Design review of the part built by this model. Coordinates are the model's own, in mm. A direction names the side the tool comes from. Give positions to 0.01 mm unless a question says otherwise; leave off trailing zeros. Order: outer loops, then holes, each group sorted by start corner. A loop starts at its lowest first (then second) coordinate and runs counter-clockwise, first axis right, second up. Notation, with made-up numbers: (56.25, 20) - (64.25, 20) arc R19 ccw to (64.25, 28) - close; hole circle Ø3 at (-12, 87). An arc over 180 degrees is marked (long way). Write each question's results on one line, items separated by ' | '. Start each with the question number.
```python
from build123d import *

# Parameters (mm, degrees)
F0_W        = 29.464
F0_H        = 43.434
F1_DEPTH    = 25.4
F2_T1_DEPTH = 50.8
F3_R        = 5.08


# Not quite as in the source:
# - a fillet or chamfer that OpenCascade refuses, or shapes differently, is made with other operations: its cross-section is extruded or revolved along the edge and cut away or added


with BuildPart() as f1:
    # F0 (on Top) → F1 (new body)
    with BuildSketch(Plane.XY):
        Polygon((25.527, -26.797), (25.527, 26.797), (-25.527, 26.797), (-25.527, 0), (-20.447, 0), (-20.447, 21.717), (-14.097, 21.717), (-14.097, -26.797), align=None)
        with Locations((5.715, 0)):
            Rectangle(F0_W, F0_H, mode=Mode.SUBTRACT)
    extrude(amount=F1_DEPTH)

    # F2: fillet of radius 5.08 on 6 edges, made by hand

    # F2_s2 → F2_t1 (cut)
    with BuildSketch(Plane.XY.offset(-12.7)):
        with BuildLine():
            ThreePointArc((-20.447, 26.797), (-24.0391024484, 25.3091024484), (-25.527, 21.717))
            Line((-25.527, 21.717), (-25.527, 26.797))
            Line((-25.527, 26.797), (-20.447, 26.797))
        make_face()
        with BuildLine():
            ThreePointArc((25.527, 21.717), (24.0391024484, 25.3091024484), (20.447, 26.797))
            Line((20.447, 26.797), (25.527, 26.797))
            Line((25.527, 26.797), (25.527, 21.717))
        make_face()
        with BuildLine():
            ThreePointArc((-9.017, -26.797), (-12.6091024484, -25.3091024484), (-14.097, -21.717))
            Line((-14.097, -21.717), (-14.097, -26.797))
            Line((-14.097, -26.797), (-9.017, -26.797))
        make_face()
        with BuildLine():
            ThreePointArc((20.447, -26.797), (24.0391024484, -25.3091024484), (25.527, -21.717))
            Line((25.527, -21.717), (25.527, -26.797))
            Line((25.527, -26.797), (20.447, -26.797))
        make_face()
        with BuildLine():
            ThreePointArc((-25.527, 0), (-21.9348975516, 1.4878975516), (-20.447, 5.08))
            Line((-20.447, 5.08), (-20.447, 0))
            Line((-20.447, 0), (-25.527, 0))
        make_face()
        with BuildLine():
            ThreePointArc((-25.527, 5.08), (-24.0391024484, 1.4878975516), (-20.447, 0))
            Line((-20.447, 0), (-25.527, 0))
            Line((-25.527, 0), (-25.527, 5.08))
        make_face()
    extrude(amount=F2_T1_DEPTH, mode=Mode.SUBTRACT)

    # F3
    f3_edges = [f1.edges().sort_by_distance(p)[0] for p in [
        (-9.017, -21.717, 12.7),
        (20.447, -21.717, 12.7),
        (20.447, 21.717, 12.7),
        (-9.017, 21.717, 12.7),
    ]]
    fillet(f3_edges, radius=F3_R)


solid = f1.part
```
Q1. Add section C-C (z = 14.5). Give the boundary of the cut face in (x, y).
Q2. Add section B-B (y = 0). Give the boundary of the cut face in (x, z), plus the area to 3 significant figures.
Q3. Draft analysis for pull direction Y (two halves, no side actions). For faces 1 (the flat face through (6, -26.797, 13)), 2 (the flat face through (6, -21.717, 13)), 3 (the flat face through (-14.097, 0, 13)), 4 (the cylindrical face through (19, 20.19, 12.88)), state which applies: pulls with the +Y half, pulls with the -Y half, needs draft (parallel to the pull), parting line crosses it, or undercut.
Q4. Insertion check: pin 1 Ø7.5 at (y, z) = (-5.5, 12.5) entering from -X; pin 2 Ø2 at (x, z) = (-11.5, 11) entering from -Y; pin 3 Ø1.9 at (x, z) = (-17.5, 12) entering from -Y. Each pin has a flat end and moves straight along its axis. Give the tip position at first contact, or say it passes through.
Q5. Add section A-A (x = 2.5). Give the boundary of the cut face in (y, z), plus the area to 3 significant figures.
Q6. Add section D-D (y = 18). Give the boundary of the cut face in (x, z), plus the area to 3 significant figures.
Q7. For line 1 (X direction, y = 12, z = 6.25); line 2 (Y direction, x = 5.5, z = 16.75); line 3 (X direction, y = 20, z = 8.75), list the stretches that pass through material, from the lowest coordinate up. Write a range as [from, to].
Q8. Machinability: for faces 5 (the flat face through (-17, 21.717, 13)), 6 (the flat face through (20.447, 0, 13)), 7 (the cylindrical face through (-12.57, -25.35, 12.52)), which of the approach directions +Z, -Z, +X, -X, +Y, -Y give a long, thin tool a straight path to every point of the face, cutting with its end or side? Answer none if there is none.
Verdict:
1) outline: (-25.53, 5.08) arc R5.08 ccw to (-22.99, 0.68) arc R5.08 ccw to (-20.45, 5.08) - (-20.45, 21.72) - (-14.1, 21.72) - (-14.1, -21.72) arc R5.08 ccw to (-9.02, -26.8) - (20.45, -26.8) arc R5.08 ccw to (25.53, -21.72) - (25.53, 21.72) arc R5.08 ccw to (20.45, 26.8) - (-20.45, 26.8) arc R5.08 ccw to (-25.53, 21.72) - close; hole (-9.02, -16.64) arc R5.08 ccw to (-3.94, -21.72) - (15.37, -21.72) arc R5.08 ccw to (20.45, -16.64) - (20.45, 16.64) arc R5.08 ccw to (15.37, 21.72) - (-3.94, 21.72) arc R5.08 ccw to (-9.02, 16.64) - close
2) outline: (-14.1, 0) - (-9.02, 0) - (-9.02, 25.4) - (-14.1, 25.4) - close; (20.45, 0) - (25.53, 0) - (25.53, 25.4) - (20.45, 25.4) - close | area: 258 mm2
3) face 1: pulls with the -Y half | face 2: undercut | face 3: needs draft | face 4: undercut
4) pin 1: stops at x = -14.1 | pin 2: stops at y = -26.58 | pin 3: stops at y = 21.72
5) outline: (-26.8, 0) - (-21.72, 0) - (-21.72, 25.4) - (-26.8, 25.4) - close; (21.72, 0) - (26.8, 0) - (26.8, 25.4) - (21.72, 25.4) - close | area: 258 mm2
6) outline: (-25.53, 0) - (-20.45, 0) - (-20.45, 25.4) - (-25.53, 25.4) - close; (-14.1, 0) - (-8.83, 0) - (-8.83, 25.4) - (-14.1, 25.4) - close; (20.26, 0) - (25.53, 0) - (25.53, 25.4) - (20.26, 25.4) - close | area: 397 mm2
7) line 1: x = [-25.53, -20.45], [-14.1, -9.02], [20.45, 25.53] | line 2: y = [-26.8, -21.72], [21.72, 26.8] | line 3: x = [-25.53, -20.45], [-14.1, -7.74], [19.17, 25.53]
8) face 5: +Z, -Z, -Y | face 6: +Z, -Z | face 7: +Z, -Z, -X, -Y
